Part model, mm, in its own coordinate system. A direction names the side the tool comes from. Coordinates: 2 decimals unless noted, no trailing zeros. Loops run counter-clockwise (first coordinate to the right, second up) from the corner with the lowest first, then second, coordinate; pieces in that order, holes last. Notation, with made-up numbers: (39, 32.25) -> (53, 32.25) arc R19 cw to (53, 53.25) -> close; hole circle Ø9 at (88, 23.25). An arc over 180 degrees is marked (long way). One line per question, with ' | ' between items. Start each with the question number.
1) Probe L1, parallel to Z at x = 55.95, y = 5.2; L2, parallel to Z at x = 0, y = -0.25; L3, parallel to X at y = 5.35, z = -15. List the from-to ranges inside material, lowest first. Write a range as from..to.
2) Cut at D-D (x = 19). List the corners of the cut face in (y, z), plus the area to 3 significant figures.
3) Cut at A-A (x = -3). Count the separate pieces of the cut face and the enclosed holes in it, plus the area to 3 significant figures.
4) Drop flat-ended pins along their axis: pin 1 (4.5 mm diameter, centred on x = -18, y = 1.5, fed in from +Z); pin 2 (2.5 mm diameter, centred on x = 52, y = 1, fed in from +Z); pin 3 (2.5 mm diameter, centred on x = 55.95, z = -15, fed in from +Y); pin 4 (10 mm diameter, centred on x = 38, z = 1.5, fed in from -Y). Give the stop position or say it passes through.
5) 3-axis set-ups, long thin cutter, end or side, ignore diameter. For faces 4 (the face through (42, 1, 17)), 5 (the face through (-12, 1.57, 21.02)), 6 (the face through (40, -2.5, 0)), 7 (the face through (-5, -1, 5)), 8 (the face through (45, 1, -20)): which of +Z, -Z, +X, -X, +Y, -Y reach the whole face in a straight line?
6) Two-plate mould, pull along X, no slides. Class faces 1 (the face through (22, 1, -18)), 2 (the face through (15, 7, -14)), 3 (the face through (40, 5.5, 0)): released by +X, released by -X, zero draft, split by the parting line, or undercut.
7) Cut at B-B (z = -7). List the corners of the cut face in (x, y).
8) Cut at C-C (y = -3.5). List the corners of the cut face in (x, z).
from build123d import *

# Parameters (mm, degrees)
BOSS_EXTRUDE1_DEPTH             = 5
BOSS_EXTRUDE1_DEPTH_BACK        = 5
SHELL1_T                        = -3
BOSS_EXTRUDE2_START             = 5
BOSS_EXTRUDE2_DEPTH             = 3
SKETCH2_R                       = 1.5
CUT_EXTRUDE1_DEPTH              = 100
F_1_4_20_TAPPED_HOLE1_D         = 5.1054
SKETCH9_W                       = 40
SKETCH9_H                       = 2.5
CUT_EXTRUDE2_DEPTH              = 79.072082078
SKETCH10_W                      = 10
SKETCH10_H                      = 45
CUT_EXTRUDE3_DEPTH              = 2.5
CUT_EXTRUDE4_START              = -10.5
SKETCH10_2_W                    = 10
SKETCH10_2_H                    = 45
CUT_EXTRUDE4_DEPTH              = 2.5
F_2_0MM_CLEARANCE_DOWEL_HOLE2_D = 2


with BuildPart() as part:
    # Sketch1 → Boss-Extrude1 (new, two sides: drawn at the far end of the back side and taken through both)
    with BuildSketch(Plane(origin=(0, 0, 0), x_dir=(1, 0, 0), z_dir=(0, 1, 0)).offset(-BOSS_EXTRUDE1_DEPTH_BACK)):
        Polygon((-25, -5), (-25, -22.5), (25, -22.5), (25, -20), (65, -20), (65, 20), (25, 20), (25, 22.5), (-25, 22.5), (-25, 5), (15, 5), (15, -5), align=None)
    extrude(amount=BOSS_EXTRUDE1_DEPTH + BOSS_EXTRUDE1_DEPTH_BACK)

    # Shell1
    shell1_openings = [part.faces().sort_by_distance(p)[0] for p in [
        (21.449275362, 5, 0),
    ]]
    offset(amount=SHELL1_T, openings=shell1_openings, kind=Kind.INTERSECTION)

    # Sketch1<2> → Boss-Extrude2 (add)
    with BuildSketch(Plane(origin=(0, 0, 0), x_dir=(1, 0, 0), z_dir=(0, 1, 0)).offset(BOSS_EXTRUDE2_START)):
        Polygon((-25, -5), (-25, -22.5), (25, -22.5), (25, -20), (65, -20), (65, 20), (25, 20), (25, 22.5), (-25, 22.5), (-25, 5), (15, 5), (15, -5), align=None)
    extrude(amount=BOSS_EXTRUDE2_DEPTH)

    # Sketch2 → Cut-Extrude1 (cut)
    with BuildSketch(Plane.XY.offset(22.5)):
        with Locations((-10.5, 1.5)):
            Circle(SKETCH2_R)
    extrude(amount=-CUT_EXTRUDE1_DEPTH, mode=Mode.SUBTRACT)

    # 1/4-20 Tapped Hole1 (through all)
    with Locations(Plane.XY.offset(22.5)):
        with Locations((-3, 1.5), (-18, 1.5)):
            Hole(F_1_4_20_TAPPED_HOLE1_D / 2)

    # Sketch9 → Cut-Extrude2 (cut, through all)
    with BuildSketch(Plane.XY.offset(20)):
        with Locations((45, 6.75)):
            Rectangle(SKETCH9_W, SKETCH9_H)
        with Locations((45, -3.75)):
            Rectangle(SKETCH9_W, SKETCH9_H)
    extrude(amount=-CUT_EXTRUDE2_DEPTH, mode=Mode.SUBTRACT)

    # Sketch10 → Cut-Extrude3 (cut)
    with BuildSketch(Plane(origin=(0, 8, 0), x_dir=(1, 0, 0), z_dir=(0, 1, 0))):
        with Locations((20, 0)):
            Rectangle(SKETCH10_W, SKETCH10_H)
    extrude(amount=-CUT_EXTRUDE3_DEPTH, mode=Mode.SUBTRACT)

    # Sketch10<2> → Cut-Extrude4 (cut)
    with BuildSketch(Plane(origin=(0, 8, 0), x_dir=(1, 0, 0), z_dir=(0, 1, 0)).offset(CUT_EXTRUDE4_START)):
        with Locations((20, 0)):
            Rectangle(SKETCH10_2_W, SKETCH10_2_H)
    extrude(amount=-CUT_EXTRUDE4_DEPTH, mode=Mode.SUBTRACT)

    # Ø2.0mm Clearance Dowel Hole2 (through all)
    with Locations(Plane(origin=(0, 5.5, 0), x_dir=(1, 0, 0), z_dir=(0, 1, 0))):
        with Locations((31.950000364, 15), (31.950000364, -15), (55.950000364, -15), (55.950000364, 15)):
            Hole(F_2_0MM_CLEARANCE_DOWEL_HOLE2_D / 2)


solid = part.part
Reported:
1) L1: z = -20..-16, -14..14, 16..20 | L2: z = -22.5..-19.5, -8..-5, 5..8, 19.5..22.5 | L3: x = -25..30.95, 32.95..54.95, 56.95..65
2) outline: (-2.5, -22.5) -> (5.5, -22.5) -> (5.5, 22.5) -> (-2.5, 22.5) -> close; hole (-2, -19.5) -> (5, -19.5) -> (5, 19.5) -> (-2, 19.5) -> close | area: 87.0 mm²
3) separate pieces: 4 | enclosed holes: 0 | area: 233 mm²
4) pin 1: passes through | pin 2: stops at z = 20 | pin 3: stops at y = 5.5 | pin 4: stops at y = -2.5
5) face 4: none | face 5: +Z, -Z | face 6: +Z, -Z, +X, -Y | face 7: -X, +Y, -Y | face 8: -Z, +X, +Y, -Y
6) face 1: undercut | face 2: released by +X | face 3: zero draft
7) outline: (-25, -5) -> (15, -5) -> (15, -2.5) -> (65, -2.5) -> (65, 5.5) -> (15, 5.5) -> (15, 8) -> (-25, 8) -> close; hole circle Ø5.11 at (-18, 1.5); hole circle Ø3 at (-10.5, 1.5); hole circle Ø5.11 at (-3, 1.5); hole (18, -2) -> (62, -2) -> (62, 5) -> (18, 5) -> close
8) outline: (-25, -22.5) -> (15, -22.5) -> (15, -5) -> (-25, -5) -> close; (-25, 5) -> (15, 5) -> (15, 22.5) -> (-25, 22.5) -> close
